The listing builds one solid part. Answer for the finished solid, in the listing's coordinates (mm). Give positions to 0.01 mm unless a question says otherwise; leave off trailing zeros. Write each loop counter-clockwise with the first axis right and the second up, starting at its lowest first coordinate (ties: lowest second). Pieces come first, ordered by that corner, then holes. Notation, with made-up numbers: M 79.5,-30 L 105.5,-30 A23 cw 105.5,4 Z; hole C 43,-33.5 d7. An arc over 180 degrees is marked long. Answer as a JSON object with one key per item and string values.
Autodesk Inventor part; units mm, degrees
ref_plane "YZ Plane" through (0, 0, 0) normal (1, 0, 0) x (0, 1, 0)
ref_plane "XZ Plane" through (0, 0, 0) normal (0, 1, 0) x (-1, 0, 0)
ref_plane "XY Plane" through (0, 0, 0) normal (0, 0, 1) x (1, 0, 0)
sketch "Sketch1" plane through (0, 0, 0) normal (0, 1, 0) x (-1, 0, 0)
  circle A0 centre (0, 0) radius 10
  dimension "d0" = 20
extrude "Extrusion1" add sketch "Sketch1" along normal blind 610
sketch "Sketch2" plane through (0, 610, 0) normal (0, 1, 0) x (1, 0, 0)
  circle A0 centre (0, 0) radius 20
  dimension "d3" = 40
extrude "Extrusion2" add sketch "Sketch2" along normal blind 20
fillet "Fillet1" radius 20 1 edges at (-20, 630, 0)
sketch "Sketch3" plane through (0, 0, 0) normal (0, 0, 1) x (1, 0, 0)
  line L0 (20, 610) -> (-20, 610)
  line L1 (-20, 610) -> (20, 610)
  line L2 (20, 610) -> (20, 469.6128)
  line L3 (20, 469.6128) -> (-20, 469.6128)
  line L4 (-20, 469.6128) -> (-20, 610)
  point P0 (0, 0)
split_face "Split1"
sketch "Sketch4" plane through (0, 0, 0) normal (0, 0, 1) x (1, 0, 0)
  line L0 (0, 0) -> (27.9883, 0)
  line L1 (27.9883, 0) -> (27.9883, 20.3959)
  line L2 (27.9883, 20.3959) -> (-23.698, 20.3959)
  line L3 (-23.698, 20.3959) -> (-23.698, 0)
  line L4 (-23.698, 0) -> (27.9883, 0)
split_face "Split2"
sketch "Sketch5" plane through (0, 0, 0) normal (0, 0, 1) x (1, 0, 0)
  line L0 (10, 469.6128) -> (-10, 469.6128)
  line L1 (-6.0106, 469.6128) -> (-6.0106, 612.6424)
  line L2 (-6.0106, 612.6424) -> (-55.0341, 605.0239)
  line L3 (-55.0341, 605.0239) -> (-35.491, 440.7287)
  line L4 (-35.491, 440.7287) -> (-6.0106, 469.6128)
  point P0 (0, 0)
split_face "Split3"
properties part number "Haste Contrapeso" material "Steel, Carbon"
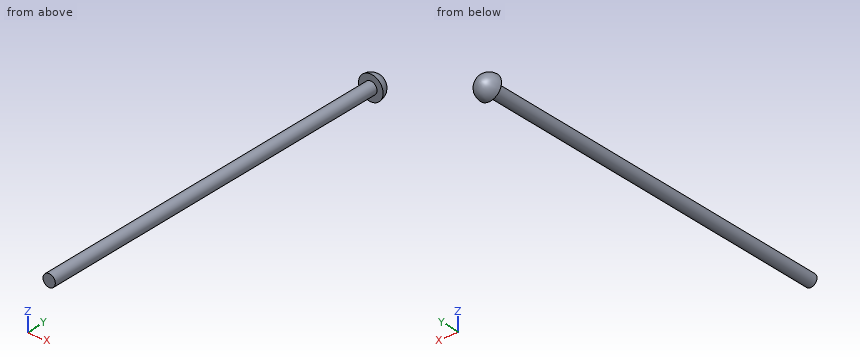
1. Flat-ended cylindrical pins translate along their axes: pin 1 (5 mm diameter, centred on x = 9, z = -13.5, fed in from +Y); pin 2 (5 mm diameter, centred on x = 14, z = -8, fed in from -Y); pin 3 (3 mm diameter, centred on y = 551.5, z = -5, fed in from +X). Find the tip coordinate at first contact, or state that the pin passes through.
Verdict:
{"pin 1": "stops at y = 624.55", "pin 2": "stops at y = 610", "pin 3": "stops at x = 9.37"}
2. A cutting plane is placed at A-A, the plane y = 479.5. Give the vertices of the cut face in (x, z), plus the area to 3 significant figures.
Verdict:
{"outline": "C 0,0 d20", "area": "314 mm2"}
3. Consider line 1 along X through (y, z) = (457.5, 1); line 2 along X through (y, z) = (327.5, -0.5); line 3 along Y through (x, z) = (-11, -14.5). Determine where each line is inside the solid, lowest interval first.
Verdict:
{"line 1": "x = -9.95 to 9.95", "line 2": "x = -9.99 to 9.99", "line 3": "y = 610 to 618.29"}
